Geometry: final body of the model. Coordinates: model frame, mm. Face numbers are marked on the shaded views. A direction names the side the tool comes from. Round coordinates to 2 decimals unless told otherwise and drop trailing zeros. Write each loop counter-clockwise with the first axis right and the second up, starting at its lowest first coordinate (ties: lowest second). Pieces come first, ordered by that corner, then holes. Notation, with made-up numbers: (88.25, -29.5) -> (142.25, -29.5) arc R29 ccw to (142.25, -9.5) -> close; hole circle Ø2 at (25.25, 20). An arc over 180 degrees is marked (long way). One line per item, written item: value. Start each with the question number.
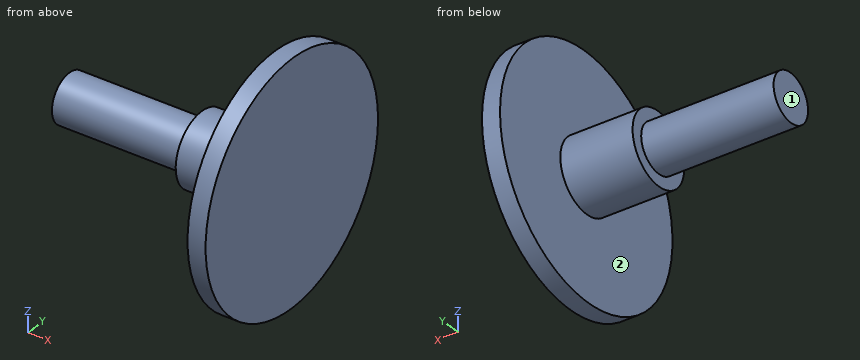
from build123d import *

# Parameters (mm, degrees)
SKETCH_2_R      = 3
EXTRUDE_1_DEPTH = 6


with BuildPart() as part:
    # 草图1 → 旋转1 (revolve)
    with BuildSketch(Plane.XY):
        Polygon((-18.5, 0), (-18.5, 2), (-1.5, 2), (-1.5, 10), (0, 10), (0, 2), (0, 0), align=None)
    revolve(axis=Axis((-18.5, 0, 0), (1, 0, 0)))

    # 草图2 → 凸台-拉伸1 (add)
    with BuildSketch(Plane.ZY.offset(1.5)):
        Circle(SKETCH_2_R)
    extrude(amount=EXTRUDE_1_DEPTH)


solid = part.part
(1) Line query: probe 1 along X at (y, z) = (3.75, -2); probe 2 along Z at (x, y) = (-1, -0.5); probe 3 along Y at (x, z) = (-17, -0.25). Output: solid intervals per line, ascending.
(2) Section query A-A (z = 0). Output: boundary loops of the cut face in (x, y).
(3) Section query D-D (x = -5.5). Output: boundary loops of the cut face in (y, z).
(4) Set-up query: the marked faces 1 and 2. Return all of +Z, -Z, +X, -X, +Y, -Y with unobstructed straight access to the full face (end or side cutting, diameter ignored); none if empty.
(5) Section query C-C (x = -16.75). Output: boundary loops of the cut face in (y, z).
(6) Pin query (flat end, axial travel): pin 1 (1 mm diameter, centred on y = -4, z = -4, fed in from -X); pin 2 (2 mm diameter, centred on y = -5, z = 4, fed in from +X); pin 3 (10 mm diameter, centred on x = -16.5, z = -3.5, fed in from -Y); pin 4 (4 mm diameter, centred on x = -11.5, y = 1.5, fed in from -Z). Return the tip coordinate at first contact, or that it passes through.
Results list:
1. probe 1: x = -1.5 to 0
1. probe 2: z = -9.99 to 9.99
1. probe 3: y = -1.98 to 1.98
2. outline: (-18.5, -2) -> (-7.5, -2) -> (-7.5, -3) -> (-1.5, -3) -> (-1.5, -10) -> (0, -10) -> (0, 10) -> (-1.5, 10) -> (-1.5, 3) -> (-7.5, 3) -> (-7.5, 2) -> (-18.5, 2) -> close
3. outline: circle Ø6 at (0, 0)
4. face 1: +Z, -Z, -X, +Y, -Y
4. face 2: -X
5. outline: circle Ø4 at (0, 0)
6. pin 1: stops at x = -1.5
6. pin 2: stops at x = 0
6. pin 3: stops at y = -2
6. pin 4: stops at z = -2
